Geometry check sheet. Reference: the model listing, model coordinates, mm. Round coordinates to 2 decimals unless told otherwise and drop trailing zeros. Order: outer loops, then holes, each group sorted by start corner. A loop starts at its lowest first (then second) coordinate and runs counter-clockwise, first axis right, second up.
```python
from build123d import *

# Parameters (mm, degrees)
SKETCH14_W              = 3.9751
SKETCH14_H              = 31.75
CUT_EXTRUDE10_START     = -10.379628209
CUT_EXTRUDE10_DEPTH     = 20.759256418
CUT_EXTRUDE9_DEPTH      = 34.872578542
CUT_EXTRUDE9_DEPTH_BACK = 34.872578542
SKETCH17_R              = 8.016875
CUT_EXTRUDE4_DEPTH      = 35.562321428
CUT_EXTRUDE4_DEPTH_BACK = 35.562321428
SKETCH10_R              = 3.96875
CUT_EXTRUDE7_START      = -5.55625
SKETCH22_W              = 22.225
SKETCH22_H              = 26.9875
CUT_EXTRUDE7_DEPTH      = 30.006071428
CUT_EXTRUDE8_START      = 5.55625
SKETCH23_W              = 22.225
SKETCH23_H              = 26.9875
CUT_EXTRUDE8_DEPTH      = 30.006071428
CHAMFER1_SIZE           = 1.05918
CHAMFER2_SIZE           = 0.396875


# Read off the part's stored shape, not the designer's step: Cut-Extrude10
with BuildPart() as part:
    # Sketch14 → Revolve4 (revolve)
    with BuildSketch(Plane.XY, mode=Mode.PRIVATE) as revolve4_sk:
        with Locations((1.98755, -15.875)):
            Rectangle(SKETCH14_W, SKETCH14_H)
    revolve(revolve4_sk.sketch.rotate(Axis((0, 0, 0), (0, -1, 0)), 180), axis=Axis((0, 0, 0), (0, -1, 0)))

    # Chamfer1
    chamfer1_edges = [part.edges().sort_by_distance(p)[0] for p in [
        (3.9751, -31.75, 0),
    ]]
    chamfer(chamfer1_edges, length=CHAMFER1_SIZE)


with BuildPart() as body_2:
    # Sketch21 → Revolve5 (revolve)
    with BuildSketch(Plane.XY):
        with BuildLine():
            Line((0, 26.9875), (0, 0))
            Line((0, 0), (3.9751, 0))
            ThreePointArc((3.9751, 0), (4.86426259, 4.14604002), (7.37536085, 7.562857762))
            ThreePointArc((7.37536085, 7.562857762), (10.388848273, 19.819551662), (0, 26.9875))
        make_face()
    revolve(axis=Axis((0, 0, 0), (0, -1, 0)))

    # Cut-Extrude10 outline → Cut-Extrude10 (cut)
    with BuildSketch(Plane(origin=(0, 0, 0), x_dir=(0, 0, -1), z_dir=(1, 0, 0)).offset(CUT_EXTRUDE10_START)):
        Polygon((-3.9911, -2), (-3.96875, 0.79375), (-3.96875, 28), (-12, 28), (-12, -2), align=None)
        Polygon((3.96875, 0.79375), (3.9911, -2), (12, -2), (12, 28), (3.96875, 28), align=None)
    extrude(amount=CUT_EXTRUDE10_DEPTH, mode=Mode.SUBTRACT)

    # Sketch17 → Cut-Extrude9 (cut, two sides: drawn at the far end of the back side and taken through both)
    with BuildSketch(Plane.XY.offset(-CUT_EXTRUDE9_DEPTH_BACK)):
        with Locations(Location((0, 15.875, 0), (0, 0, 270))):
            Circle(SKETCH17_R)
    extrude(amount=CUT_EXTRUDE9_DEPTH + CUT_EXTRUDE9_DEPTH_BACK, mode=Mode.SUBTRACT)

    # Combine2: union part
    add(part.part)


with BuildPart() as body_3:
    # Sketch7 → Revolve3 (revolve)
    with BuildSketch(Plane.XY):
        with BuildLine():
            Line((0, 23.8125), (0, 7.9375))
            ThreePointArc((0, 7.9375), (7.9375, 15.875), (0, 23.8125))
        make_face()
    revolve(axis=Axis((0, 0, 0), (0, 1, 0)))

    # Sketch10 → Cut-Extrude4 (cut, two sides: drawn at the far end of the back side and taken through both)
    with BuildSketch(Plane.XY.offset(-CUT_EXTRUDE4_DEPTH_BACK)):
        with Locations(Location((0, 15.875, 0), (0, 0, 180))):
            Circle(SKETCH10_R)
    extrude(amount=CUT_EXTRUDE4_DEPTH + CUT_EXTRUDE4_DEPTH_BACK, mode=Mode.SUBTRACT)

    # Sketch22 → Cut-Extrude7 (cut, through all)
    with BuildSketch(Plane.XY.offset(CUT_EXTRUDE7_START)):
        with Locations((0, 13.49375)):
            Rectangle(SKETCH22_W, SKETCH22_H)
    extrude(amount=-CUT_EXTRUDE7_DEPTH, mode=Mode.SUBTRACT)

    # Sketch23 → Cut-Extrude8 (cut, through all)
    with BuildSketch(Plane.XY.offset(CUT_EXTRUDE8_START)):
        with Locations((0, 13.49375)):
            Rectangle(SKETCH23_W, SKETCH23_H)
    extrude(amount=CUT_EXTRUDE8_DEPTH, mode=Mode.SUBTRACT)

    # Chamfer2
    chamfer2_edges = [body_3.edges().sort_by_distance(p)[0] for p in [
        (3.96875, 15.875, -5.55625),
        (3.96875, 15.875, 5.55625),
    ]]
    chamfer(chamfer2_edges, length=CHAMFER2_SIZE)


solid = body_2.part
```
(1) Draft check along X on faces 1 (the cylindrical face through (0.352, 23.884, -0.056)), 2 (the flat face through (0, -31.75, 0)), 3 (the cylindrical face through (0.86, -15.13, 3.88)). Enter one of: released by +X, released by -X, zero draft, split by the parting line, or undercut.
Returned:
face 1: undercut
face 2: zero draft
face 3: split by the parting line
(2) Sectioned sample at B-B, the plane y = 18. Record the cut outline in (x, z), and give its area (3 significant figures).
Returned:
outline: (-10.16, -3.97) - (-7.73, -3.97) - (-7.73, 3.97) - (-10.16, 3.97) arc R10.91 ccw to start; (7.73, -3.97) - (10.16, -3.97) arc R10.91 ccw to (10.16, 3.97) - (7.73, 3.97) - close
area: 46.5 mm2
(3) Sectioned sample at C-C, the plane y = -13.5. Record the cut outline in (x, z).
Returned:
outline: circle Ø7.95 at (0, 0)
(4) Material ranges on line 1 (Y direction, x = 0, z = -2); line 2 (Y direction, x = 0, z = 0.5); line 3 (Z direction, x = 9, y = 17), recorded low to high.
Returned:
line 1: y = -31.75 to 7.86, 23.89 to 26.81
line 2: y = -31.75 to 7.86, 23.89 to 26.98
line 3: z = -3.97 to 3.97
(5) Sectioned sample at D-D, the plane x = -9.5. Record the cut outline in (y, z) (3 decimals), and give its area (3 significant figures).
Returned:
outline: (11.693, -3.969) - (20.057, -3.969) arc R5.765 ccw to (20.057, 3.969) - (11.693, 3.969) arc R5.765 ccw to start
area: 83.7 mm2
(6) Depth check by flat-ended pin: P1, Ø3, axis at x = -5.5, z = -1.5, coming from the +Y side; P2, Ø6, axis at x = 2.5, y = 10, coming from the -Z side; P3, Ø1.5, axis at x = 7.5, z = 3, coming from the -Y side. Enter the tip coordinate at first touch or a pass-through.
Returned:
P1: stops at y = 26.16
P2: stops at z = -3.97
P3: stops at y = 7.52
